from build123d import *

# Parameters (mm, degrees)
SKETCH_1_R               = 18
EXTRUDE_1_DEPTH          = 65
FILLET_1_R               = 18
CUT_EXTRUDE_2_DEPTH      = 70.806876452
CUT_EXTRUDE_2_DEPTH_BACK = 70.806876452
SKETCH_2_OUTSIDE_W       = 54.514
SKETCH_2_OUTSIDE_H       = 83.514
SKETCH_3_R               = 6
CUT_EXTRUDE_3_DEPTH      = 80
M12X1_75_1_D             = 10.2
M12X1_75_1_DEPTH         = 32.75
M12X1_75_1_TIP           = 3.064389157
FILLET_2_R               = 1


with BuildPart() as part:
    # 草图1 → 拉伸1 (new body)
    with BuildSketch(Plane(origin=(0, 0, 0), x_dir=(1, 0, 0), z_dir=(0, 1, 0))):
        with Locations(Location((0, 0, 0), (0, 0, 270))):
            Circle(SKETCH_1_R)
    extrude(amount=EXTRUDE_1_DEPTH)

    # 圆角1
    fillet_1_edges = [part.edges().sort_by_distance(p)[0] for p in [
        (0, 65, -18),
    ]]
    fillet(fillet_1_edges, radius=FILLET_1_R)

    # 草图2 outside → 拉伸2 (cut, two sides: drawn at the far end of the back side and taken through both)
    with BuildSketch(Plane.XY.offset(-CUT_EXTRUDE_2_DEPTH_BACK)):
        with Locations((0, 32.5)):
            Rectangle(SKETCH_2_OUTSIDE_W, SKETCH_2_OUTSIDE_H)
        Polygon((-12.5, 0), (-12.5, 15), (-10, 15), (-10, 85.518474484), (10, 85.518474484), (10, 15), (12.5, 15), (12.5, 0), align=None, mode=Mode.SUBTRACT)
    extrude(amount=CUT_EXTRUDE_2_DEPTH + CUT_EXTRUDE_2_DEPTH_BACK, mode=Mode.SUBTRACT)

    # 草图3 → 拉伸3 (cut)
    with BuildSketch(Plane.ZY.offset(10)):
        with Locations((0, 47)):
            Circle(SKETCH_3_R)
    extrude(amount=-CUT_EXTRUDE_3_DEPTH, mode=Mode.SUBTRACT)

    # M12x1.75 螺纹孔1
    with Locations(Plane.XZ):
        with Locations((0, 0)):
            Hole(M12X1_75_1_D / 2, depth=M12X1_75_1_DEPTH)
            with Locations((0, 0, -(M12X1_75_1_DEPTH + M12X1_75_1_TIP / 2))):  # 118° drill point
                Cone(0, M12X1_75_1_D / 2, M12X1_75_1_TIP, mode=Mode.SUBTRACT)

    # 圆角2
    fillet_2_edges = [part.edges().sort_by_distance(p)[0] for p in [
        (-10, 31, -14.966629547),
        (-10, 31, 14.966629547),
        (10, 31, 14.966629547),
        (10, 31, -14.966629547),
        (10, 61.966629547, 0),
        (-10, 61.966629547, 0),
    ]]
    fillet(fillet_2_edges, radius=FILLET_2_R)


solid = part.part
Can you work these out from the model? Positions are in its coordinate system, mm. A direction names the side the tool comes from. Coordinates: 2 decimals unless noted, no trailing zeros. Loops run counter-clockwise (first coordinate to the right, second up) from the corner with the lowest first, then second, coordinate; pieces in that order, holes last. Notation, with made-up numbers: (80.5, 31) - (106.5, 31) arc R21 cw to (106.5, 43) - close; hole circle Ø10 at (54, 12.5). An arc over 180 degrees is marked (long way). Put each result on its own line as item: value. Start each with the question number.
Item 1: Suppose I cut it at B-B (x = -7.5). Please give me the cut outline in (y, z).
Item 2: For pin 1 (19 mm diameter, centred on y = 47, z = 0, fed in from +X); pin 2 (8.5 mm diameter, centred on y = 37.5, z = -2, fed in from -X); pin 3 (2 mm diameter, centred on x = -2, y = 12, fed in from -Z); pin 4 (3 mm diameter, centred on x = 4.5, z = -3.5, fed in from -Y), each with a flat end and sliding along its axis, tell me the tip position at first contact or that it passes through.
Item 3: If we mould it in two halves opening along Y, with no side actions, what happens to faces 1 (the face through (6, 0, 0)), 2 (the face through (-10, 38, 0)), 3 (the face through (-0.14, 41.143, -1.301))? For each: +Y half, -Y half, draft (parallel to the pull), parting line (faces both ways), or undercut.
Item 4: Suppose I cut it at A-A (y = 29.5). Please give me the cut outline in (x, z), and give its area (3 significant figures).
Item 5: Which directions (+Z, -Z, +X, -X, +Y, -Y) give clear straight access to the entire face, cutting with the end or side of a thin tool? Please do faces 4 (the face through (-2.4, 16.6, -4.5)), 5 (the face through (10, 39, 0)), 6 (the face through (12.5, 8, 0)).
Item 6: If I drill on line 1 along Z through (x, y) = (0, 17.5); line 2 along X through (y, z) = (18, 0); line 3 along Y through (x, z) = (7.5, 1), over which ranges is the centre line in solid material (lowest first)?
Here are the results:
1. outline: (0, -16.36) - (47, -16.36) arc R16.36 ccw to (47, 16.36) - (0, 16.36) - close; hole circle Ø12 at (47, 0)
2. pin 1: x = 10
2. pin 2: x = -10
2. pin 3: z = -17.97
2. pin 4: y = 0
3. face 1: -Y half
3. face 2: draft
3. face 3: undercut
4. outline: (-10, -14.42) arc R1 ccw to (-9.53, -15.27) arc R18 ccw to (9.53, -15.27) arc R1 ccw to (10, -14.42) - (10, 14.42) arc R1 ccw to (9.53, 15.27) arc R18 ccw to (-9.53, 15.27) arc R1 ccw to (-10, 14.42) - close; hole circle Ø10.2 at (0, 0)
4. area: 599 mm²
5. face 4: -Y
5. face 5: +Z, -Z, +X, +Y
5. face 6: +Z, -Z, +X, +Y, -Y
6. line 1: -18 to -5.1, 5.1 to 18
6. line 2: -10 to -5.1, 5.1 to 10
6. line 3: 0 to 41.08, 52.92 to 63.33
